Check sheet for the modelled part. Datum: model origin and axes. Units: mm. Face numbers are marked on the shaded views. A direction names the side the tool comes from. Give positions to 0.01 mm unless a question says otherwise; leave off trailing zeros. Order: outer loops, then holes, each group sorted by start corner. A loop starts at its lowest first (then second) coordinate and runs counter-clockwise, first axis right, second up. Notation, with made-up numbers: (-5, 18) -> (49, 18) arc R26 ccw to (49, 52) -> close; hole circle Ø7 at (85.25, 35). An arc over 180 degrees is marked (long way). Answer in a Markdown table with one row per item. Add a question column.
(1) Cross-section at B-B (y = 4). Record the cut outline in (x, z).
(2) Cross-section at A-A (x = 38.5). Record the cut outline in (y, z), then the cut area to 3 significant figures.
(3) Cross-section at D-D (z = 27.5). Record the cut outline in (x, y).
(4) Release check for a two-part mould opening along Y. For the marked faces 1, 2 and 3 record: released by +Y, released by -Y, zero draft, split by the parting line, or undercut.
(5) Go/stop test with flat-tipped pins: pin 1 (0.8 mm diameter, centred on x = 16, z = 5, fed in from +Y); pin 2 (3 mm diameter, centred on y = 10, z = 52, fed in from -X); pin 3 (1.1 mm diameter, centred on x = 31, z = 31, fed in from +Y). Record where each tip stops, or that it passes through.
(6) Thickness scan on L1, parallel to Z at x = 11, y = 4.75; L2, parallel to X at y = 8.5, z = 13; L3, parallel to Y at x = 8.5, z = 32. Record the ranges inside material, lowest first. Write a range as [from, to].
(7) Set-up check for the marked faces 4 and 5: record each of +Z, -Z, +X, -X, +Y, -Y from which the full face is reachable in a straight line by a thin tool's end or side.
(8) Cross-section at C-C (x = 44). Record the cut outline in (y, z), then the cut area to 3 significant figures.
```python
from build123d import *

# Parameters (mm, degrees)
SKETCH1_W           = 47
SKETCH1_H           = 55.5
BOSS_EXTRUDE1_DEPTH = 15
CUT_EXTRUDE4_DEPTH  = 54
FILLET1_R           = 7
FILLET2_R           = 7
SKETCH3_W           = 4.401923789
SKETCH3_H           = 6.5
CUT_EXTRUDE5_DEPTH  = 54
SKETCH4_W           = 1
SKETCH4_H           = 1
CUT_EXTRUDE6_DEPTH  = 54
CUT_EXTRUDE7_DEPTH  = 20
CUT_EXTRUDE8_DEPTH  = 5
BOSS_EXTRUDE3_DEPTH = 1.5


with BuildPart() as part:
    # Sketch1 → Boss-Extrude1 (new body)
    with BuildSketch(Plane(origin=(0, 0, 0), x_dir=(1, 0, 0), z_dir=(0, 1, 0))):
        with Locations((23.5, -27.75)):
            Rectangle(SKETCH1_W, SKETCH1_H)
    extrude(amount=BOSS_EXTRUDE1_DEPTH)

    # Sketch2 → Cut-Extrude4 (cut)
    with BuildSketch(Plane.XY.offset(55.5)):
        with BuildLine():
            ThreePointArc((11.098076211, 15), (8.5, 15.5), (5.901923789, 15))
            Line((5.901923789, 15), (11.098076211, 15))
        make_face()
        with BuildLine():
            Line((11.098076211, 15), (5.901923789, 15))
            ThreePointArc((5.901923789, 15), (4.574858823, 2.70403013), (15.5, 8.5))
            ThreePointArc((15.5, 8.5), (14.29596987, 12.425141177), (11.098076211, 15))
        make_face()
        with BuildLine():
            ThreePointArc((26.098076211, 15), (23.5, 15.5), (20.901923789, 15))
            Line((20.901923789, 15), (26.098076211, 15))
        make_face()
        with BuildLine():
            Line((26.098076211, 15), (20.901923789, 15))
            ThreePointArc((20.901923789, 15), (19.574858823, 2.70403013), (30.5, 8.5))
            ThreePointArc((30.5, 8.5), (29.29596987, 12.425141177), (26.098076211, 15))
        make_face()
        with BuildLine():
            ThreePointArc((45.5, 8.5), (44.29596987, 12.425141177), (41.098076211, 15))
            Line((41.098076211, 15), (35.901923789, 15))
            ThreePointArc((35.901923789, 15), (34.574858823, 2.70403013), (45.5, 8.5))
        make_face()
        with BuildLine():
            Line((35.901923789, 15), (41.098076211, 15))
            ThreePointArc((41.098076211, 15), (38.5, 15.5), (35.901923789, 15))
        make_face()
    extrude(amount=-CUT_EXTRUDE4_DEPTH, mode=Mode.SUBTRACT)

    # Fillet1
    fillet1_edges = [part.edges().sort_by_distance(p)[0] for p in [
        (47, 15, 27.75),
    ]]
    fillet(fillet1_edges, radius=FILLET1_R)

    # Fillet2
    fillet2_edges = [part.edges().sort_by_distance(p)[0] for p in [
        (0, 15, 27.75),
    ]]
    fillet(fillet2_edges, radius=FILLET2_R)

    # Sketch3 → Cut-Extrude5 (cut)
    with BuildSketch(Plane.XY.offset(55.5)):
        with Locations((28.299038106, 11.75)):
            Rectangle(SKETCH3_W, SKETCH3_H)
        with Locations((33.700961895, 11.75)):
            Rectangle(SKETCH3_W, SKETCH3_H)
        with Locations((13.299038106, 11.75)):
            Rectangle(SKETCH3_W, SKETCH3_H)
        with Locations((18.700961895, 11.75)):
            Rectangle(SKETCH3_W, SKETCH3_H)
    extrude(amount=-CUT_EXTRUDE5_DEPTH, mode=Mode.SUBTRACT)

    # Sketch4 → Cut-Extrude6 (cut)
    with BuildSketch(Plane.XY.offset(55.5)):
        with Locations((16, 14.5)):
            Rectangle(SKETCH4_W, SKETCH4_H)
        with Locations((31, 14.5)):
            Rectangle(SKETCH4_W, SKETCH4_H)
    extrude(amount=-CUT_EXTRUDE6_DEPTH, mode=Mode.SUBTRACT)

    # Sketch5 → Cut-Extrude7 (cut)
    with BuildSketch(Plane.ZY.offset(-15.5)):
        Polygon((6.5, 14), (50.5, 14), (40.5, 7), (16.5, 7), align=None)
    extrude(amount=-CUT_EXTRUDE7_DEPTH, mode=Mode.SUBTRACT)

    # Sketch5_2 → Cut-Extrude8 (cut)
    with BuildSketch(Plane.ZY.offset(-15.5)):
        Polygon((6.5, 14), (50.5, 14), (40.5, 7), (16.5, 7), align=None)
    extrude(amount=CUT_EXTRUDE8_DEPTH, mode=Mode.SUBTRACT)

    # Sketch6 → Boss-Extrude3 (add)
    with BuildSketch(Plane.XY.offset(55.5)):
        with BuildLine():
            Line((0, 0), (47, 0))
            Line((47, 0), (47, 8))
            ThreePointArc((47, 8), (44.949747468, 12.949747468), (40, 15))
            Line((40, 15), (7, 15))
            ThreePointArc((7, 15), (2.050252532, 12.949747468), (0, 8))
            Line((0, 8), (0, 0))
        make_face()
    extrude(amount=BOSS_EXTRUDE3_DEPTH)


solid = part.part
```
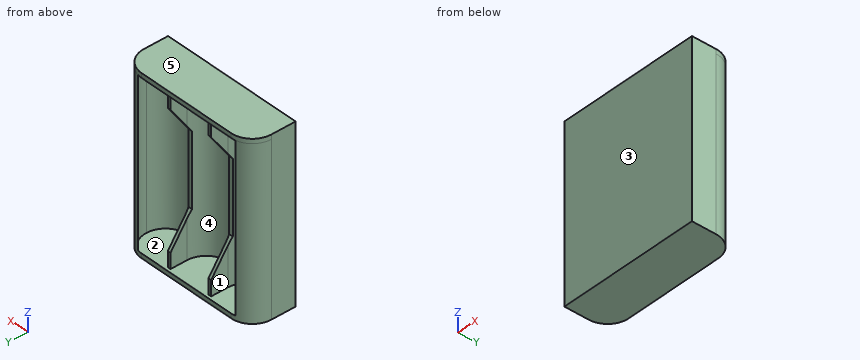
Answer below:
| question | item | result |
|---|---|---|
| 1 | outline | (0, 0) -> (47, 0) -> (47, 57) -> (0, 57) -> close; hole (3.14, 1.5) -> (13.86, 1.5) -> (13.86, 55.5) -> (3.14, 55.5) -> close; hole (18.14, 1.5) -> (28.86, 1.5) -> (28.86, 55.5) -> (18.14, 55.5) -> close; hole (33.14, 1.5) -> (43.86, 1.5) -> (43.86, 55.5) -> (33.14, 55.5) -> close |
| 2 | outline | (0, 0) -> (15, 0) -> (15, 1.5) -> (1.5, 1.5) -> (1.5, 55.5) -> (15, 55.5) -> (15, 57) -> (0, 57) -> close |
| 2 | area | 126 mm² |
| 3 | outline | (0, 0) -> (47, 0) -> (47, 8) arc R7 ccw to (41.45, 14.85) arc R7 cw (long way) to (31.66, 7) -> (30.34, 7) arc R7 cw to (16.66, 7) -> (15.34, 7) arc R7 cw (long way) to (5.55, 14.85) arc R7 ccw to (0, 8) -> close |
| 4 | face 1 | zero draft |
| 4 | face 2 | undercut |
| 4 | face 3 | released by -Y |
| 5 | pin 1 | stops at y = 14 |
| 5 | pin 2 | stops at x = 0.02 |
| 5 | pin 3 | stops at y = 7 |
| 6 | L1 | z = [0, 1.5], [55.5, 57] |
| 6 | L2 | x = [0.02, 1.5], [15.5, 16.5], [30.5, 31.5], [45.5, 46.98] |
| 6 | L3 | y = [0, 1.5] |
| 7 | face 4 | +Y |
| 7 | face 5 | +Z, +X, -X, +Y, -Y |
| 8 | outline | (0, 0) -> (13.74, 0) -> (13.74, 57) -> (0, 57) -> close; hole (4.17, 1.5) -> (12.83, 1.5) -> (12.83, 55.5) -> (4.17, 55.5) -> close |
| 8 | area | 316 mm² |
